Verification items for the finished model (mm, model axes). Face numbers are marked on the shaded views. A direction names the side the tool comes from. Coordinates: 2 decimals unless noted, no trailing zeros. Write each loop counter-clockwise with the first axis right and the second up, starting at its lowest first coordinate (ties: lowest second). Pieces come first, ordered by that corner, then holes. Notation, with made-up numbers: M -32,80.25 L 5,80.25 A16 ccw 5,86.25 Z; hole C -20.5,68 d6. An arc over 180 degrees is marked long. One line per item, written item: value.
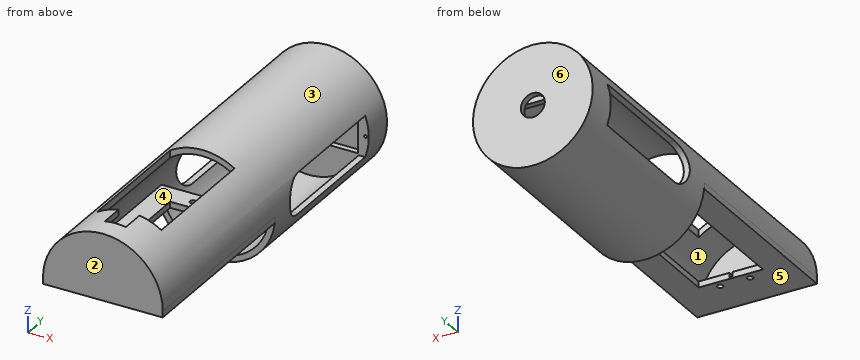
```python
from build123d import *

# Parameters (mm, degrees)
SKETCH1_R           = 20
SKETCH1_R_2         = 18
BOSS_EXTRUDE1_DEPTH = 65
SKETCH2_R           = 18
BOSS_EXTRUDE2_DEPTH = 2
SKETCH4_W           = 24.70942711
SKETCH4_H           = 65
CUT_EXTRUDE1_DEPTH  = 79.89866919
SKETCH5_W           = 39.998874984
SKETCH5_H           = 65
BOSS_EXTRUDE3_DEPTH = 2
SKETCH6_W           = 21.5
SKETCH6_H           = 42.3
CUT_EXTRUDE2_DEPTH  = 72.523580028
SKETCH7_R           = 1
CUT_EXTRUDE3_DEPTH  = 2
SKETCH8_W           = 1
SKETCH8_H           = 55
CUT_EXTRUDE4_DEPTH  = 1.5
BOSS_EXTRUDE4_START = -2.4
SKETCH9_R           = 18
BOSS_EXTRUDE4_DEPTH = 2.4
CUT_EXTRUDE5_DEPTH  = 79.89866919
SKETCH11_R          = 18.596328204
SKETCH11_W          = 22.6
SKETCH11_H          = 12.5
BOSS_EXTRUDE6_DEPTH = 2
SKETCH12_R          = 0.5
CUT_EXTRUDE6_DEPTH  = 3
SKETCH15_R          = 4
CUT_EXTRUDE8_DEPTH  = 5
SKETCH16_R          = 20
CUT_EXTRUDE9_DEPTH  = 0.4
SKETCH18_W          = 7
SKETCH18_H          = 8
CUT_EXTRUDE10_DEPTH = 71.929701261


with BuildPart() as part:
    # Sketch1 → Boss-Extrude1 (new, symmetric)
    with BuildSketch(Plane(origin=(0, 0, 0), x_dir=(1, 0, 0), z_dir=(0, 1, 0))):
        with Locations(Location((0, 0, 0), (0, 0, 270))):
            Circle(SKETCH1_R)
        with Locations(Location((0, 0, 0), (0, 0, 270))):
            Circle(SKETCH1_R_2, mode=Mode.SUBTRACT)
    extrude(amount=BOSS_EXTRUDE1_DEPTH, both=True)

    # Sketch2 → Boss-Extrude2 (add)
    with BuildSketch(Plane.XZ.offset(65)):
        with Locations(Location((0, 0, 0), (0, 0, 270))):
            Circle(SKETCH2_R)
    extrude(amount=-BOSS_EXTRUDE2_DEPTH)

    # Sketch4 → Cut-Extrude1 (cut, through all)
    with BuildSketch(Plane(origin=(20, 0, 0), x_dir=(0, 0, -1), z_dir=(1, 0, 0))):
        with Locations((12.504713555, -32.5)):
            Rectangle(SKETCH4_W, SKETCH4_H)
    extrude(amount=-CUT_EXTRUDE1_DEPTH, mode=Mode.SUBTRACT)

    # Sketch5 → Boss-Extrude3 (add)
    with BuildSketch(Plane(origin=(0, 0, -0.15), x_dir=(-1, 0, 0), z_dir=(0, 0, -1))):
        with Locations((0, -32.5)):
            Rectangle(SKETCH5_W, SKETCH5_H)
    extrude(amount=BOSS_EXTRUDE3_DEPTH)

    # Sketch6 → Cut-Extrude2 (cut, through all)
    with BuildSketch(Plane(origin=(0, 0, -2.15), x_dir=(-1, 0, 0), z_dir=(0, 0, -1))):
        with Locations((0, -28.65)):
            Rectangle(SKETCH6_W, SKETCH6_H)
    extrude(amount=-CUT_EXTRUDE2_DEPTH, mode=Mode.SUBTRACT)

    # Sketch7 → Cut-Extrude3 (cut)
    with BuildSketch(Plane(origin=(0, 0, -2.15), x_dir=(-1, 0, 0), z_dir=(0, 0, -1))):
        with Locations((-5, -4.3)):
            Circle(SKETCH7_R)
        with Locations((-5, -52.3)):
            Circle(SKETCH7_R)
        with Locations(Location((5, -52.3, 0), (0, 0, 180))):
            Circle(SKETCH7_R)
        with Locations(Location((5, -4.3, 0), (0, 0, 180))):
            Circle(SKETCH7_R)
    extrude(amount=-CUT_EXTRUDE3_DEPTH, mode=Mode.SUBTRACT)

    # Sketch8 → Cut-Extrude4 (cut)
    with BuildSketch(Plane.XY.offset(-0.15)):
        with Locations((0, -28.3)):
            Rectangle(SKETCH8_W, SKETCH8_H)
    extrude(amount=-CUT_EXTRUDE4_DEPTH, mode=Mode.SUBTRACT)

    # Sketch9 → Boss-Extrude4 (add)
    with BuildSketch(Plane(origin=(0, 65, 0), x_dir=(1, 0, 0), z_dir=(0, 1, 0)).offset(BOSS_EXTRUDE4_START)):
        with Locations(Location((0, 0, 0), (0, 0, 6.860040985))):
            Circle(SKETCH9_R)
    extrude(amount=BOSS_EXTRUDE4_DEPTH)

    # Sketch10 → Cut-Extrude5 (cut, through all)
    with BuildSketch(Plane(origin=(20, 0, 0), x_dir=(0, 0, -1), z_dir=(1, 0, 0))):
        with BuildLine():
            Line((-6.85, 54.1), (6.85, 54.1))
            Line((6.85, 54.1), (6.85, 15.35))
            ThreePointArc((6.85, 15.35), (0, 8.5), (-6.85, 15.35))
            Line((-6.85, 15.35), (-6.85, 54.1))
        make_face()
    extrude(amount=-CUT_EXTRUDE5_DEPTH, mode=Mode.SUBTRACT)

    # Sketch11 → Boss-Extrude6 (add)
    with BuildSketch(Plane.XZ.offset(-54.1)):
        Circle(SKETCH11_R)
        with Locations((5.1, 0)):
            Rectangle(SKETCH11_W, SKETCH11_H, mode=Mode.SUBTRACT)
    extrude(amount=-BOSS_EXTRUDE6_DEPTH)

    # Sketch12 → Cut-Extrude6 (cut)
    with BuildSketch(Plane.XZ.offset(-54.1)):
        with Locations(Location((18.9, 0, 0), (0, 0, 270))):
            Circle(SKETCH12_R)
        with Locations(Location((-8.7, 0, 0), (0, 0, 270))):
            Circle(SKETCH12_R)
    extrude(amount=-CUT_EXTRUDE6_DEPTH, mode=Mode.SUBTRACT)

    # Sketch15 → Cut-Extrude8 (cut)
    with BuildSketch(Plane(origin=(0, 65, 0), x_dir=(1, 0, 0), z_dir=(0, 1, 0))):
        with Locations(Location((0, 0, 0), (0, 0, 270))):
            Circle(SKETCH15_R)
    extrude(amount=-CUT_EXTRUDE8_DEPTH, mode=Mode.SUBTRACT)

    # Sketch16 → Cut-Extrude9 (cut)
    with BuildSketch(Plane(origin=(0, 65, 0), x_dir=(1, 0, 0), z_dir=(0, 1, 0))):
        with Locations(Location((0, 0, 0), (0, 0, 6.171221478))):
            Circle(SKETCH16_R)
    extrude(amount=-CUT_EXTRUDE9_DEPTH, mode=Mode.SUBTRACT)

    # Sketch18 → Cut-Extrude10 (cut, through all)
    with BuildSketch(Plane.XY.offset(-0.15)):
        with Locations((0, -53.8)):
            Rectangle(SKETCH18_W, SKETCH18_H)
    extrude(amount=CUT_EXTRUDE10_DEPTH, mode=Mode.SUBTRACT)


solid = part.part
```
Item 1: Scan lines: line 1 (Y direction, x = 5.5, z = 8); line 2 (X direction, y = 55, z = 0); line 3 (Y direction, x = 0, z = 5.5). Record each from-to range of solid material in increasing order.
The answers:
line 1: y = -65 to -63, 54.1 to 56.1, 62.6 to 64.6
line 2: x = -20 to -9.2, -8.2 to -6.2, 16.4 to 18.4, 19.4 to 20
line 3: y = -65 to -63, 62.6 to 64.6
Item 2: Go/stop test with flat-tipped pins: P1, Ø3, axis at x = 5, y = -4.3, coming from the -Z side; P2, Ø2.5, axis at x = 5, y = -52.3, coming from the +Z side; P3, Ø8, axis at x = 8.5, y = 47, coming from the +Z side; P4, Ø12, axis at y = 14, z = 0, coming from the +X side. Record where each tip stops, or that it passes through.
The answers:
P1: stops at z = -2.15
P2: stops at z = 19.65
P3: stops at z = 19.49
P4: stops at x = 20
Item 3: Draft check along X on the marked faces 1, 2 and 3. Enter one of: released by +X, released by -X, zero draft, split by the parting line, or undercut.
The answers:
face 1: undercut
face 2: zero draft
face 3: split by the parting line
Item 4: Cross-section at D-D, the plane z = 12. Enter the section's corners in (x, y), and give its area (3 significant figures).
The answers:
outline: M -16,-65 L 16,-65 L 16,64.6 L -16,64.6 Z; hole M -13.42,-63 L 13.42,-63 L 13.42,54.1 L -13.42,54.1 Z; hole M -13.42,56.1 L 13.42,56.1 L 13.42,62.6 L -13.42,62.6 Z
area: 831 mm²
Item 5: Cross-section at B-B, the plane x = -2. Give the number of separate pieces and of enclosed holes in the cut face, and give its area (3 significant figures).
The answers:
separate pieces: 4
enclosed holes: 0
area: 475 mm²
Item 6: Cross-section at C-C, the plane y = 6. Enter the section's corners in (x, z), and give its area (3 significant figures).
The answers:
outline: C 0,0 d40; hole C 0,0 d36
area: 239 mm²
Item 7: Cross-section at A-A, the plane y = 27. Enter the section's corners in (x, z).
The answers:
outline: M -18.79,-6.85 A20 ccw 18.79,-6.85 L 16.65,-6.85 A18 cw -16.65,-6.85 Z; M -18.79,6.85 L -16.65,6.85 A18 cw 16.65,6.85 L 18.79,6.85 A20 ccw Z
Item 8: Access from +Z, -Z, +X, -X, +Y, -Y to the whole of each face (thin tool, end or side, straight path). Record for the marked faces 4, 5 and 6.
The answers:
face 4: none
face 5: -Z, +X, -X, -Y
face 6: +Z, -Z, +X, -X, +Y
